```python
from build123d import *

# Parameters (mm, degrees)
BOSS_EXTRU_1_DEPTH      = 11.5
ENL_V_MAT_EXTRU_1_DEPTH = 7.5


with BuildPart() as part:
    # Esquisse1 → Boss.-Extru.1 (new body)
    with BuildSketch(Plane.XY):
        with BuildLine():
            Line((-11, 0), (11, 0))
            Line((11, 0), (11, 22))
            ThreePointArc((11, 22), (0, 33), (-11, 22))
            Line((-11, 22), (-11, 0))
        make_face()
    extrude(amount=BOSS_EXTRU_1_DEPTH)

    # Esquisse2 → Enlèv. mat.-Extru.1 (cut)
    with BuildSketch(Plane.XY.offset(11.5)):
        with BuildLine():
            Line((-10, 1), (-10, 22))
            ThreePointArc((-10, 22), (0, 32), (10, 22))
            Line((10, 22), (10, 1))
            Line((10, 1), (-10, 1))
        make_face()
    extrude(amount=-ENL_V_MAT_EXTRU_1_DEPTH, mode=Mode.SUBTRACT)


solid = part.part
```
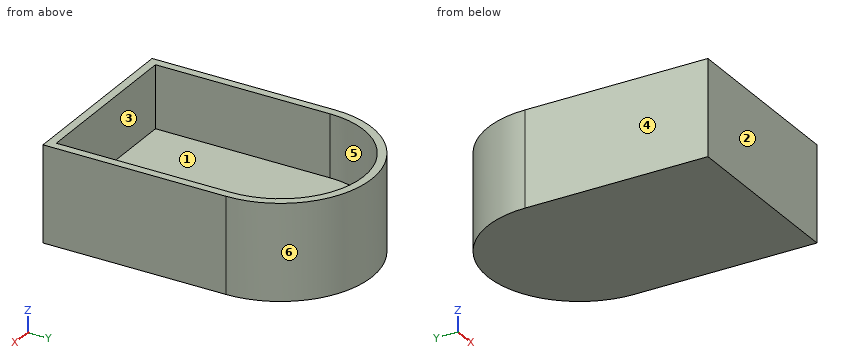
CAD build for the part. Positions are in the model's coordinates, mm. Face numbers are marked on the shaded views. A direction names the side the tool comes from. Coordinates: 2 decimals unless noted, no trailing zeros. Order: outer loops, then holes, each group sorted by start corner. A loop starts at its lowest first (then second) coordinate and runs counter-clockwise, first axis right, second up. Notation, with made-up numbers: (2.25, 2.25) -> (9.25, 2.25) arc R28 cw to (9.25, 24.25) -> close; hole circle Ø4 at (-29.5, -34.75). An arc over 180 degrees is marked (long way). Use one line per item in the form item = value. Start each with the question number.
1) Drop flat-ended pins along their axis: pin 1 (1.5 mm diameter, centred on x = 3, y = 13.5, fed in from +Z); pin 2 (4 mm diameter, centred on y = 28, z = 10, fed in from +X). Give the stop position or say it passes through.
2) Band-saw the part on D-D on z = 2.5. Give the cut face in (x, y).
3) Pull direction X, two halves, no side cores. Call the marked faces 1, 2, 3 and 4: +X half, -X half, draft (parallel to the pull), parting line (faces both ways), or undercut.
4) Band-saw the part on C-C on y = 23.5. Give the cut face in (x, z).
5) Band-saw the part on A-A on z = 7.5. Give the cut face in (x, y).
6) Drill centre lines: L1, parallel to X at y = 19, z = 5.5; L2, parallel to Z at x = -3, y = 14; L3, parallel to X at y = 28.5, z = 11. Where is each one in solid material? Low to high. Write a range as [from, to].
7) Band-saw the part on B-B on x = 0. Give the cut face in (y, z), then the cut area to 3 significant figures.
8) Tool access for the marked faces 5 and 6: list every direction of +Z, -Z, +X, -X, +Y, -Y with a clear straight run to the whole face (end or side of a thin tool).
Entries:
q1.pin_1 = 4
q1.pin_2 = 10.25
q2.outline = (-11, 0) -> (11, 0) -> (11, 22) arc R11 ccw to (-11, 22) -> close
q3.face_1 = undercut
q3.face_2 = draft
q3.face_3 = undercut
q3.face_4 = -X half
q4.outline = (-10.9, 0) -> (10.9, 0) -> (10.9, 11.5) -> (9.89, 11.5) -> (9.89, 4) -> (-9.89, 4) -> (-9.89, 11.5) -> (-10.9, 11.5) -> close
q5.outline = (-11, 0) -> (11, 0) -> (11, 22) arc R11 ccw to (-11, 22) -> close; hole (-10, 1) -> (10, 1) -> (10, 22) arc R10 ccw to (-10, 22) -> close
q6.L1 = [-11, -10], [10, 11]
q6.L2 = [0, 4]
q6.L3 = [-8.87, -7.6], [7.6, 8.87]
q7.outline = (0, 0) -> (33, 0) -> (33, 11.5) -> (32, 11.5) -> (32, 4) -> (1, 4) -> (1, 11.5) -> (0, 11.5) -> close
q7.area = 147 mm2
q8.face_5 = +Z
q8.face_6 = +Z, -Z, +Y
